Could you check a few things on this model? Use its own coordinates, in mm. Coordinates: 2 decimals unless noted, no trailing zeros. Loops run counter-clockwise (first coordinate to the right, second up) from the corner with the lowest first, then second, coordinate; pieces in that order, holes last. Notation, with made-up numbers: M 12.5,85 L 22.5,85 A33 ccw 22.5,122 Z; hole C -12.5,4.25 d3. An arc over 180 degrees is marked long. Write each question's results on one line, items separated by ' | '.
```python
from build123d import *

# Parameters (mm, degrees)
ESBO_O1_R                = 1.143
ESBO_O1_R_2              = 2.819211747
RESSALTO_EXTRUS_O1_DEPTH = 1.65


with BuildPart() as part:
    # Esboço1 → Ressalto-extrusão1 (new body)
    with BuildSketch(Plane.XY):
        with BuildLine():
            ThreePointArc((-4.302124406, -4.182311163), (-4.077931794, -4.401189993), (-3.842618859, -4.608066989))
            ThreePointArc((-3.842618859, -4.608066989), (0, -6.000000089), (3.842618859, -4.608066989))
            ThreePointArc((3.842618859, -4.608066989), (4.074890318, -4.404006128), (4.296341713, -4.188251301))
            ThreePointArc((4.296341713, -4.188251301), (5.607085842, -3.223218185), (7.158341274, -2.730322991))
            ThreePointArc((7.158341274, -2.730322991), (9.52094015, 0), (7.158341274, 2.730322991))
            ThreePointArc((7.158341274, 2.730322991), (5.607085842, 3.223218185), (4.296341713, 4.188251301))
            ThreePointArc((4.296341713, 4.188251301), (4.077931794, 4.401189993), (3.848982033, 4.602753348))
            ThreePointArc((3.848982033, 4.602753348), (0.008290039, 5.999994362), (-3.836248349, 4.613371834))
            ThreePointArc((-3.836248349, 4.613371834), (-4.074890318, 4.404006128), (-4.302124406, 4.182311163))
            ThreePointArc((-4.302124406, 4.182311163), (-5.593565523, 3.224698333), (-7.12215689, 2.726450484))
            ThreePointArc((-7.12215689, 2.726450484), (-9.458939648, 0), (-7.12215689, -2.726450484))
            ThreePointArc((-7.12215689, -2.726450484), (-5.593565523, -3.224698333), (-4.302124406, -4.182311163))
        make_face()
        with Locations((6.76200015, 0)):
            Circle(ESBO_O1_R, mode=Mode.SUBTRACT)
        with Locations((-6.69999985, 0)):
            Circle(ESBO_O1_R, mode=Mode.SUBTRACT)
        Circle(ESBO_O1_R_2, mode=Mode.SUBTRACT)
    extrude(amount=RESSALTO_EXTRUS_O1_DEPTH)


solid = part.part
```
(1) Imagine slicing it at A-A, the plane y = 0. List the corners of the cut face in (x, z) for me (3 decimals).
Reported:
outline: M -9.459,0 L -7.843,0 L -7.843,1.65 L -9.459,1.65 Z; M -5.557,0 L -2.819,0 L -2.819,1.65 L -5.557,1.65 Z; M 2.819,0 L 5.619,0 L 5.619,1.65 L 2.819,1.65 Z; M 7.905,0 L 9.521,0 L 9.521,1.65 L 7.905,1.65 Z
(2) Imagine slicing it at D-D, the plane x = 6. List the corners of the cut face in (y, z) for me, and give its area (3 significant figures).
Reported:
outline: M -3.04,0 L -0.85,0 L -0.85,1.65 L -3.04,1.65 Z; M 0.85,0 L 3.04,0 L 3.04,1.65 L 0.85,1.65 Z | area: 7.23 mm2
(3) Please list where these lines run through material, in increasing order: probe 1 along Y at (x, z) = (0, 0.75); probe 2 along X at (y, z) = (1, 1.4); probe 3 along X at (y, z) = (-0.5, 1.4). Write a range as from..to.
Reported:
probe 1: y = -6..-2.82, 2.82..6 | probe 2: x = -9.27..-7.25, -6.15..-2.64, 2.64..6.21, 7.32..9.33 | probe 3: x = -9.41..-7.73, -5.67..-2.77, 2.77..5.73, 7.79..9.48
(4) If we mould it in two halves opening along Y, with no side actions, what happens to faces 1 (the cylindrical face through (-0.611, -2.752, 0.813)), 2 (the cylindrical face through (5.63, 3.21, 0.81)), 3 (the cylindrical face through (5.59, -3.23, 0.81))? For each: released by +Y, released by -Y, zero draft, split by the parting line, or undercut.
Reported:
face 1: undercut | face 2: released by +Y | face 3: released by -Y
(5) Will this pin go through, and if not, where does the flat tip stop? P1, Ø1.8, axis at x = -6.7, y = 0, coming from the -Z side.
Reported:
P1: passes through
(6) Imagine slicing it at B-B, the plane x = -6.7. List the corners of the cut face in (y, z) for me.
Reported:
outline: M -2.81,0 L -1.14,0 L -1.14,1.65 L -2.81,1.65 Z; M 1.14,0 L 2.81,0 L 2.81,1.65 L 1.14,1.65 Z
(7) Imagine slicing it at C-C, the plane z = 0.65. List the corners of the cut face in (x, y) for me (3 decimals), and give its area (3 significant figures).
Reported:
outline: M -7.122,-2.726 A5 cw -4.302,-4.182 A6 ccw 4.296,-4.188 A5 cw 7.158,-2.73 A2.759 ccw 7.158,2.73 A5 cw 4.296,4.188 A6 ccw -4.302,4.182 A5 cw -7.122,2.726 A2.759 ccw Z; hole C -6.7,0 d2.286; hole C 0,0 d5.638; hole C 6.762,0 d2.286 | area: 117 mm2
